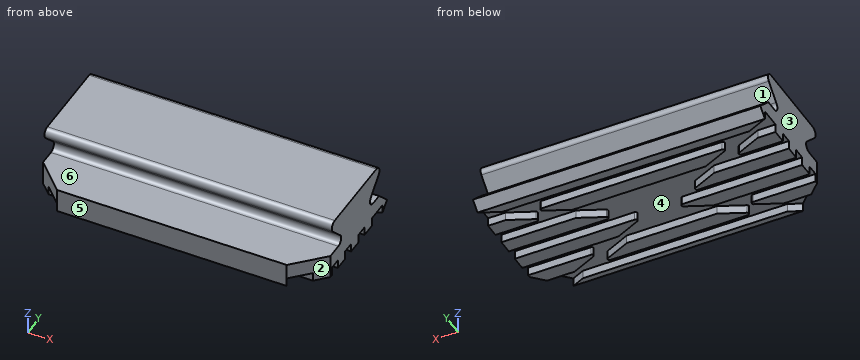
from build123d import *

# Parameters (mm, degrees)
EXTRUDE_1_DEPTH     = 49.8
CHAMFER_1_SIZE      = 5
CUT_EXTRUDE_1_DEPTH = 49.8
CUT_EXTRUDE_2_DEPTH = 1.5
CUT_EXTRUDE_5_DEPTH = 1.5
CUT_EXTRUDE_6_DEPTH = 1.5
FILLET_1_R          = 0.3


with BuildPart() as part:
    # 草图1 → 凸台-拉伸1 (new body)
    with BuildSketch(Plane(origin=(0, 0, 0), x_dir=(0, 0, -1), z_dir=(1, 0, 0))):
        with BuildLine():
            Line((-3.3011643203984544, 4.869061466212711), (-14.311631849697747, 4.869061466212711))
            Line((-14.311631849697747, 4.869061466212711), (-14.311631849697747, -2.159184752168928))
            ThreePointArc((-14.311631849697747, -2.1591847521689282), (-13.694314644696359, -3.083064362059199), (-12.60452430575002, -2.8662900962872895))
            Line((-12.60452430575002, -2.8662900962872895), (-10.135977537233877, -0.4266270598954794))
            ThreePointArc((-10.135977537233877, -0.42662705989547856), (-10.004086660367205, -0.2658876156487018), (-9.841806105066398, -0.1358976402325789))
            ThreePointArc((-9.841806105066398, -0.1358976402325789), (-8.821917682779581, -0.09946220767270797), (-8.301164320376756, -0.9771386117116159))
            Line((-8.301164320376756, -0.9771386117116161), (-8.301164320376754, -3.01590252304511))
            Line((-8.301164320376754, -3.01590252304511), (-8.301164320376756, -8.640917781834164))
            Line((-8.301164320376756, -8.640917781834164), (-3.3011643203767598, -8.640917781834164))
            Line((-3.30116432037676, -8.640917781834164), (-3.30116432037676, 4.869061466212711))
        make_face()
        with BuildLine():
            ThreePointArc((-8.301164320376754, 10.71526154413704), (-8.821917682779581, 9.837585140098131), (-9.841806105066398, 9.874020572658003))
            ThreePointArc((-9.841806105066398, 9.874020572658003), (-10.004086660367204, 10.004010548074126), (-10.135977537233877, 10.164749992320901))
            Line((-10.135977537233877, 10.164749992320901), (-12.60452430575002, 12.604413028712713))
            ThreePointArc((-12.60452430575002, 12.604413028712713), (-13.694314644696359, 12.821187294484622), (-14.311631849697747, 11.89730768459435))
            Line((-14.311631849697747, 11.89730768459435), (-14.311631849697747, 4.869061466212711))
            Line((-14.311631849697747, 4.869061466212711), (-3.3011643203984544, 4.869061466212711))
            Line((-3.30116432037676, 4.869061466212711), (-3.30116432037676, 13.139889713283024))
            Line((-3.30116432037676, 13.139889713283026), (-5.608236006167775, 15.446957584376776))
            Line((-5.608236006167775, 15.446957584376776), (-8.301164320376754, 12.754025455470533))
            Line((-8.301164320376754, 12.754025455470533), (-8.301164320376756, 10.71526154413704))
        make_face()
    extrude(amount=EXTRUDE_1_DEPTH)

    # 倒角1
    chamfer_1_edges = [part.edges().sort_by_distance(p)[0] for p in [
        (0, -8.640917781834164, 5.801164320376758),
        (49.8, -8.640917781834164, 5.801164320376758),
    ]]
    chamfer(chamfer_1_edges, length=CHAMFER_1_SIZE)

    # 草图3 → 切除-拉伸1 (cut)
    with BuildSketch(Plane(origin=(49.8, 0, 0), x_dir=(0, 0, -1), z_dir=(1, 0, 0))):
        Polygon((-4.108236006167775, 13.94696006459702), (-3.301164320376763, 13.94696006459702), (-3.30116432037676, -8.640917781834164), (-4.108236006167774, -8.640917781834164), align=None)
    extrude(amount=-CUT_EXTRUDE_1_DEPTH, mode=Mode.SUBTRACT)

    # 草图4 → 切除-拉伸2 (cut)
    with BuildSketch(Plane(origin=(0, -4.7e-16, 4.1082360061677745), x_dir=(-1, 0, 0), z_dir=(0, 1.2e-16, -1))):
        Polygon((-49.8, -5.640917781834157), (0, -5.640917781834158), (0, -7.640917781834159), (-49.8, -7.640917781834159), align=None)
        Polygon((-49.80000000000001, -1.1409177818341574), (-1.544e-14, -1.140917781834159), (-1.544e-14, -3.140917781834159), (-49.80000000000001, -3.140917781834159), align=None)
        Polygon((-49.800000000000026, 3.359082218165842), (-3.087e-14, 3.359082218165841), (-3.087e-14, 1.3590822181658406), (-49.800000000000026, 1.3590822181658406), align=None)
        Polygon((-49.80000000000005, 7.859082218165841), (-4.631e-14, 7.859082218165839), (-4.631e-14, 5.859082218165839), (-49.80000000000005, 5.859082218165839), align=None)
        Polygon((-49.80000000000006, 12.359082218165842), (-6.174e-14, 12.35908221816584), (-6.174e-14, 10.35908221816584), (-49.80000000000006, 10.35908221816584), align=None)
    extrude(amount=-CUT_EXTRUDE_2_DEPTH, mode=Mode.SUBTRACT)

    # 草图5 → 切除-拉伸5 (cut)
    with BuildSketch(Plane(origin=(0, 0, 5.608236006167775), x_dir=(-1, 0, 0), z_dir=(0, 0, -1))):
        Polygon((0, 13.94696006459702), (-46.31009994685559, -7.1308178349785605), (-44.799999999999976, -8.640917781834164), (-6.175e-14, 11.749546738532302), align=None)
        Polygon((-49.79999999999993, 11.74954673853228), (-49.8, 13.946960064596997), (-3.489900053144389, -7.13081783497854), (-4.999999999999997, -8.640917781834142), align=None)
    extrude(amount=CUT_EXTRUDE_5_DEPTH, mode=Mode.SUBTRACT)

    # 草图6 → 切除-拉伸6 (cut)
    with BuildSketch(Plane(origin=(0, -4.7e-16, 4.1082360061677745), x_dir=(-1, 0, 0), z_dir=(0, 1.2e-16, -1))):
        Polygon((-28.321709391936835, -1.1409177818341594), (-21.478290608063137, -1.1409177818341603), (-24.89999999999999, 0.41645373502506017), align=None)
        Polygon((-17.76992020746784, 5.85908221816584), (-32.03007979253217, 5.859082218165842), (-26.53731625651111, 3.3590822181658413), (-23.26268374348888, 3.3590822181658413), align=None)
    extrude(amount=-CUT_EXTRUDE_6_DEPTH, mode=Mode.SUBTRACT)

    # 圆角1
    fillet_1_edges = [part.edges().sort_by_distance(p)[0] for p in [
        (41.252239337738956, 7.85908221816584, 4.858236006167775),
        (31.36526497290105, 3.3590822181658417, 4.858236006167775),
        (41.91705415737007, 10.359082218165842, 4.858236006167775),
        (8.547760662261016, 7.85908221816585, 4.858236006167775),
        (7.8829458426299635, 10.359082218165838, 4.858236006167775),
        (22.143105427694266, 1.3590822181658417, 4.858236006167775),
        (12.25613106285637, -3.1409177818341556, 4.858236006167775),
        (11.591316243225233, -5.640917781834158, 4.8582360061677745),
        (27.656894572305735, 1.3590822181658355, 4.858236006167775),
        (37.543868937143614, -3.1409177818341654, 4.858236006167775),
        (38.208683756774704, -5.6409177818341565, 4.8582360061677745),
        (18.434735027098903, 3.3590822181658484, 4.858236006167775),
    ]]
    fillet(fillet_1_edges, radius=FILLET_1_R)


solid = part.part
The listing builds one solid part. Answer for the finished solid, in the listing's coordinates (mm). Face numbers are marked on the shaded views. A direction names the side the tool comes from. Round coordinates to 2 decimals unless told otherwise and drop trailing zeros. Write each loop counter-clockwise with the first axis right and the second up, starting at its lowest first coordinate (ties: lowest second). Pieces come first, ordered by that corner, then holes. Notation, with made-up numbers: M -22,10 L 27,10 A16 cw 27,27 Z; hole C -4,32 d7. An arc over 180 degrees is marked long. Write each question's results on one line, items separated by ' | '. Start each with the question number.
Item 1: Find section B-B on y = 2.5. Write down the section's boundary in (x, z), and give its area (3 significant figures).
Item 2: Find section A-A on x = 28. Write down the section's boundary in (y, z), and give its area (3 significant figures).
Item 3: The mould has two halves that part along X. Classify the marked faces 1, 2, 3 and 4: +X half, -X half, draft (parallel to the pull), parting line (faces both ways), or undercut.
Item 4: Straight lines are drawn through the part: probe 1 along Y at (x, z) = (36, 5.25); probe 2 along Z at (x, y) = (22, -5); probe 3 along Z at (x, y) = (29.5, 2.5). For each, find the intervals that lie inside material, in ascending order.
Item 5: Find section C-C on z = 6.5. Write down the section's boundary in (x, y).
Item 6: Which of the six approach directions +Z, -Z, +X, -X, +Y, -Y give full straight-line access (tool end or side, diameter ignored) to the marked faces 5 and 6?
Item 7: Given pin 1 Ø1.2 at (x, z) = (1.5, 4.5) entering from +Y; pin 2 Ø0.8 at (x, z) = (3.5, 5) entering from -Y; pin 3 Ø1.7 at (x, z) = (3.5, 5) entering from -Y; pin 4 Ø1.5 at (y, z) = (-2, 10.5) entering from +X, each flat-ended and moving along its own axis, determine where each tip first touches the part or whether it passes through.
Answer block:
1) outline: M 0,5.61 L 49.8,5.61 L 49.8,14.31 L 0,14.31 Z | area: 433 mm²
2) outline: M -8.64,4.11 L -7.64,4.11 L -7.64,5.61 L -5.64,5.61 L -5.64,4.11 L -3.14,4.11 L -3.14,5.61 L 7.86,5.61 L 7.86,4.11 L 10.36,4.11 L 10.36,5.61 L 12.36,5.61 L 12.36,4.11 L 13.95,4.11 L 15.45,5.61 L 12.75,8.3 L 10.72,8.3 A1 cw 10.16,10.14 L 12.6,12.6 A1 ccw 11.9,14.31 L -2.16,14.31 A1 ccw -2.87,12.6 L -0.43,10.14 A1 cw -0.98,8.3 L -8.64,8.3 Z | area: 151 mm²
3) face 1: draft | face 2: +X half | face 3: -X half | face 4: undercut
4) probe 1: y = -8.64 to -7.64, -5.64 to -4.64, -1.14 to 1.36, 3.36 to 5.47, 7.86 to 10.36, 12.36 to 15.09 | probe 2: z = 4.11 to 8.3 | probe 3: z = 5.61 to 14.31
5) outline: M 0,-3.64 L 5,-8.64 L 44.8,-8.64 L 49.8,-3.64 L 49.8,14.56 L 0,14.56 Z
6) face 5: +Z, -Z, +X, -X, -Y | face 6: +X, -X, -Y
7) pin 1: stops at y = 14.94 | pin 2: stops at y = -5.64 | pin 3: stops at y = -7.73 | pin 4: passes through
